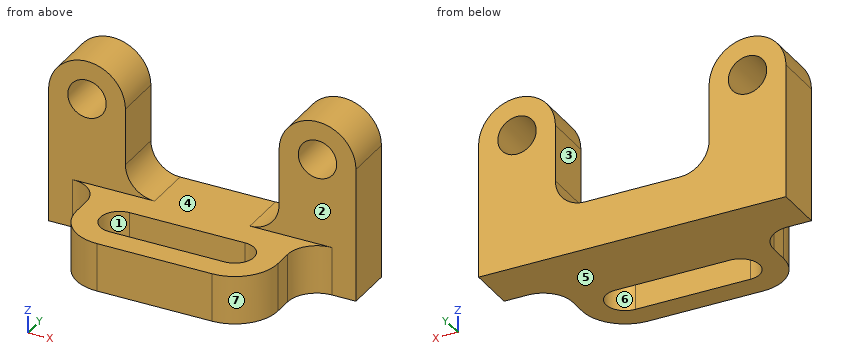
```python
from build123d import *

# Parameters (mm, degrees)
F0_R     = 6.35
F1_DEPTH = 16.002
F3_DEPTH = 29.972
F5_DEPTH = 57.151


with BuildPart() as f1:
    # F0 (on Front) → F1 (new body)
    with BuildSketch(Plane.XZ):
        with BuildLine():
            Line((0, 44.45), (0, 0))
            Line((0, 0), (101.6, 0))
            Line((101.6, 0), (101.6, 44.45))
            ThreePointArc((101.6, 44.45), (88.9, 57.15), (76.2, 44.45))
            Line((76.2, 44.45), (76.2, 25.654))
            ThreePointArc((76.2, 25.654), (73.372995, 18.829005), (66.548, 16.002))
            Line((66.548, 16.002), (35.052, 16.002))
            ThreePointArc((35.052, 16.002), (28.227005, 18.829005), (25.4, 25.654))
            Line((25.4, 25.654), (25.4, 44.45))
            ThreePointArc((25.4, 44.45), (12.7, 57.15), (0, 44.45))
        make_face()
        with Locations((12.7, 44.45)):
            Circle(F0_R, mode=Mode.SUBTRACT)
        with Locations((88.9, 44.45)):
            Circle(F0_R, mode=Mode.SUBTRACT)
    extrude(amount=F1_DEPTH)

    # F2 (on face) → F3 (join)
    with BuildSketch(Plane.XZ.offset(16.002)):
        Polygon((0, 16.002), (0, 0), (101.6, 0), (101.6, 16.002), (66.548, 16.002), (35.052, 16.002), align=None)
    extrude(amount=F3_DEPTH)

    # F4 (on face) → F5 (cut, through all)
    with BuildSketch(Plane(origin=(0, 0, 0), x_dir=(1, 0, 0), z_dir=(0, 0, -1))):
        with BuildLine():
            ThreePointArc((17.526, 31.75), (21.692113, 41.807887), (31.75, 45.974))
            Line((31.75, 45.974), (0, 45.974))
            Line((0, 45.974), (0, 16.002))
            Line((0, 16.002), (7.874, 16.002))
            ThreePointArc((7.874, 16.002), (14.698995, 18.829005), (17.526, 25.654))
            Line((17.526, 25.654), (17.526, 31.75))
        make_face()
        with BuildLine():
            Line((101.6, 45.974), (69.85, 45.974))
            ThreePointArc((69.85, 45.974), (79.907887, 41.807887), (84.074, 31.75))
            Line((84.074, 31.75), (84.074, 25.654))
            ThreePointArc((84.074, 25.654), (86.901005, 18.829005), (93.726, 16.002))
            Line((93.726, 16.002), (101.6, 16.002))
            Line((101.6, 16.002), (101.6, 45.974))
        make_face()
        with BuildLine():
            Line((69.85, 38.1), (31.75, 38.1))
            ThreePointArc((31.75, 38.1), (25.4, 31.75), (31.75, 25.4))
            Line((31.75, 25.4), (69.85, 25.4))
            ThreePointArc((69.85, 25.4), (76.2, 31.75), (69.85, 38.1))
        make_face()
    extrude(amount=-F5_DEPTH, mode=Mode.SUBTRACT)


solid = f1.part
```
Design review of the part built by this model. Coordinates are the model's own, in mm. Face numbers are marked on the shaded views. A direction names the side the tool comes from. Give positions to 0.01 mm unless a question says otherwise; leave off trailing zeros. Write each loop counter-clockwise with the first axis right and the second up, starting at its lowest first coordinate (ties: lowest second). Pieces come first, ordered by that corner, then holes. Notation, with made-up numbers: (44, 14) - (75, 14) arc R21 cw to (75, 50) - close; hole circle Ø5 at (44, -24.5). An arc over 180 degrees is marked (long way). Return JSON: item names as keys, results as strings. Group by question number.
(1) We need section D-D, the plane z = 47.5. Give the boundary of the cut face in (x, y).
(2) Machinability: for the marked faces 1, 2, 3 and 4, which of the approach directions +Z, -Z, +X, -X, +Y, -Y give a long, thin tool a straight path to every point of the face, cutting with its end or side? Answer none if there is none.
(3) We need section A-A, the plane x = 38. Give the boundary of the cut face in (y, z), then the cut area to 3 significant figures.
(4) Mouldability with a two-part tool opening along X and no side actions: class the marked faces 5, 6 and 7 as +X half, -X half, draft (parallel to the pull), parting line (faces both ways), or undercut.
(5) Insertion check: pin 1 (12 mm diameter, centred on x = 64, y = -29, fed in from +Z); pin 2 (14.5 mm diameter, centred on x = 12.7, z = 44.45, fed in from -Y); pin 3 (3 mm diameter, centred on y = -29, z = 10, fed in from -X). Each pin has a flat end and moves straight along its axis. Give the tip position at first contact, or say it passes through.
(6) To check wall thickness, follow probe 1 along X at (y, z) = (-4, 27); probe 2 along Y at (x, z) = (32, 15.5); probe 3 along X at (y, z) = (-10, 44). State the ranges of each line that lie inside material, in increasing order.
(7) We need section B-B, the plane z = 14.5. Give the boundary of the cut face in (x, y), then the cut area to 3 significant figures.
(8) We need section C-C, the plane y = -4.5. Give the boundary of the cut face in (x, z), then the cut area to 3 significant figures.
Reported:
{
 "1": {"outline": "(0.37, -16) - (7.13, -16) - (7.13, 0) - (0.37, 0) - close; (18.27, -16) - (25.03, -16) - (25.03, 0) - (18.27, 0) - close; (76.57, -16) - (83.33, -16) - (83.33, 0) - (76.57, 0) - close; (94.47, -16) - (101.23, -16) - (101.23, 0) - (94.47, 0) - close"},
 "2": {"face 1": "+Z, -Z", "face 2": "+Z, +X, -Y", "face 3": "+Z, +Y, -Y", "face 4": "+Z, -Y"},
 "3": {"outline": "(-45.97, 0) - (-38.1, 0) - (-38.1, 16) - (-45.97, 16) - close; (-25.4, 0) - (0, 0) - (0, 16) - (-25.4, 16) - close", "area": "532 mm2"},
 "4": {"face 5": "draft", "face 6": "undercut", "face 7": "+X half"},
 "5": {"pin 1": "stops at z = 16", "pin 2": "stops at y = -16", "pin 3": "stops at x = 17.53"},
 "6": {"probe 1": "x = 0 to 25.4, 76.2 to 101.6", "probe 2": "y = -45.97 to -38.1, -25.4 to 0", "probe 3": "x = 0 to 6.37, 19.03 to 25.4, 76.2 to 82.57, 95.23 to 101.6"},
 "7": {"outline": "(0, -16) - (7.87, -16) arc R9.65 cw to (17.53, -25.65) - (17.53, -31.75) arc R14.22 ccw to (31.75, -45.97) - (69.85, -45.97) arc R14.22 ccw to (84.07, -31.75) - (84.07, -25.65) arc R9.65 cw to (93.73, -16) - (101.6, -16) - (101.6, 0) - (0, 0) - close; hole (31.75, -38.1) - (69.85, -38.1) arc R6.35 ccw to (69.85, -25.4) - (31.75, -25.4) arc R6.35 ccw to start", "area": "2,960 mm2"},
 "8": {"outline": "(0, 0) - (101.6, 0) - (101.6, 44.45) arc R12.7 ccw to (76.2, 44.45) - (76.2, 25.65) arc R9.65 cw to (66.55, 16) - (35.05, 16) arc R9.65 cw to (25.4, 25.65) - (25.4, 44.45) arc R12.7 ccw to (0, 44.45) - close; hole circle Ø12.7 at (12.7, 44.45); hole circle Ø12.7 at (88.9, 44.45)", "area": "3,360 mm2"}
}
